```python
from build123d import *

# Parameters (mm, degrees)
ESBO_O1_R                = 7.5
RESSALTO_EXTRUS_O1_DEPTH = 1.2
ESBO_O2_R                = 3
RESSALTO_EXTRUS_O2_DEPTH = 7.2
ESBO_O3_R                = 4
RESSALTO_EXTRUS_O3_DEPTH = 1
ESBO_O4_R                = 3.25
ESBO_O4_R_2              = 3.0000000000000004
CORTE_EXTRUS_O1_DEPTH    = 0.5
ESBO_O5_R                = 2.5
CORTE_EXTRUS_O4_DEPTH    = 1
FILETE1_R                = 0.5


with BuildPart() as part:
    # Esboço1 → Ressalto-extrusão1 (new body)
    with BuildSketch(Plane(origin=(0, 0, 0), x_dir=(1, 0, 0), z_dir=(0, 1, 0))):
        with Locations(Location((0, 0, 0), (0, 0, 270))):
            Circle(ESBO_O1_R)
    extrude(amount=RESSALTO_EXTRUS_O1_DEPTH)

    # Esboço2 → Ressalto-extrusão2 (add)
    with BuildSketch(Plane.XZ):
        with Locations(Location((0, 0, 0), (0, 0, 90))):
            Circle(ESBO_O2_R)
    extrude(amount=RESSALTO_EXTRUS_O2_DEPTH)

    # Esboço3 → Ressalto-extrusão3 (add)
    with BuildSketch(Plane.XZ.offset(7.2)):
        with Locations(Location((0, 0, 0), (0, 0, 270))):
            Circle(ESBO_O3_R)
    extrude(amount=-RESSALTO_EXTRUS_O3_DEPTH)

    # Esboço4 → Corte-extrusão1 (cut)
    with BuildSketch(Plane(origin=(0, -6.2, 0), x_dir=(1, 0, 0), z_dir=(0, 1, 0))):
        with Locations(Location((0, 0, 0), (0, 0, 270))):
            Circle(ESBO_O4_R)
        with Locations(Location((0, 0, 0), (0, 0, 270))):
            Circle(ESBO_O4_R_2, mode=Mode.SUBTRACT)
    extrude(amount=-CORTE_EXTRUS_O1_DEPTH, mode=Mode.SUBTRACT)

    # Esboço5 → Corte-extrusão4 (cut)
    with BuildSketch(Plane.XZ.offset(7.2)):
        with Locations(Location((0, 0, 0), (0, 0, 270))):
            Circle(ESBO_O5_R)
    extrude(amount=-CORTE_EXTRUS_O4_DEPTH, mode=Mode.SUBTRACT)

    # Filete1
    # the kernel refuses this fillet: 0.5 mm, written as the material it adds along each edge
    with BuildSketch(Plane(origin=(0, -6.7, 0), x_dir=(-1.8e-16, 0, 1), z_dir=(-1, 0, -1.8e-16))) as filete1_piece_1:
        with BuildLine():
            CenterArc((3.5000000000000004, 0.4330127018922436), FILETE1_R, 180, 60.000000000001364)
            Line((3.2500000000000107, 1.865e-14), (3.0000000000000004, 0))
            Line((3.0000000000000004, 0), (3.0000000000000004, 0.4330127018922436))
        make_face()
    revolve(axis=Axis((0, -6.7, 0), (0, 1, 0)))
    with BuildSketch(Plane(origin=(0, -6.2, 0), x_dir=(-1.8e-16, 0, -1), z_dir=(-1, 0, 1.8e-16))) as filete1_piece_2:
        with BuildLine():
            CenterArc((2.5 - FILETE1_R, FILETE1_R), FILETE1_R, 270, 90)
            Line((2.5 - FILETE1_R, 0), (2.5, 0))
            Line((2.5, 0), (2.5, FILETE1_R))
        make_face()
    revolve(axis=Axis((0, -6.2, 0), (0, -1, 0)))
    # the kernel refuses this fillet: 0.5 mm, written as the material it takes off along each edge
    with BuildSketch(Plane(origin=(0, -7.2, 0), x_dir=(-1.8e-16, 0, -1), z_dir=(-1, 0, 1.8e-16))) as filete1_2_piece_1:
        with BuildLine():
            CenterArc((4 - FILETE1_R, -FILETE1_R), FILETE1_R, 0, 90)
            Line((4 - FILETE1_R, 0), (4, 0))
            Line((4, 0), (4, -FILETE1_R))
        make_face()
    revolve(axis=Axis((0, -7.2, 0), (0, -1, 0)), mode=Mode.SUBTRACT)
    with BuildSketch(Plane(origin=(0, -6.2, 0), x_dir=(-1.8e-16, 0, 1), z_dir=(-1, 0, -1.8e-16))) as filete1_2_piece_2:
        with BuildLine():
            CenterArc((3.25 + FILETE1_R, -FILETE1_R), FILETE1_R, 90, 90)
            Line((3.25 + FILETE1_R, 0), (3.25, 0))
            Line((3.25, 0), (3.25, -FILETE1_R))
        make_face()
    revolve(axis=Axis((0, -6.2, 0), (0, 1, 0)), mode=Mode.SUBTRACT)
    with BuildSketch(Plane(origin=(0, -7.2, 0), x_dir=(-1.8e-16, 0, -1), z_dir=(-1, 0, 1.8e-16))) as filete1_2_piece_3:
        with BuildLine():
            CenterArc((2.5 + FILETE1_R, -FILETE1_R), FILETE1_R, 90, 90)
            Line((2.5, -FILETE1_R), (2.5, 0))
            Line((2.5, 0), (2.5 + FILETE1_R, 0))
        make_face()
    revolve(axis=Axis((0, -7.2, 0), (0, -1, 0)), mode=Mode.SUBTRACT)


solid = part.part
```
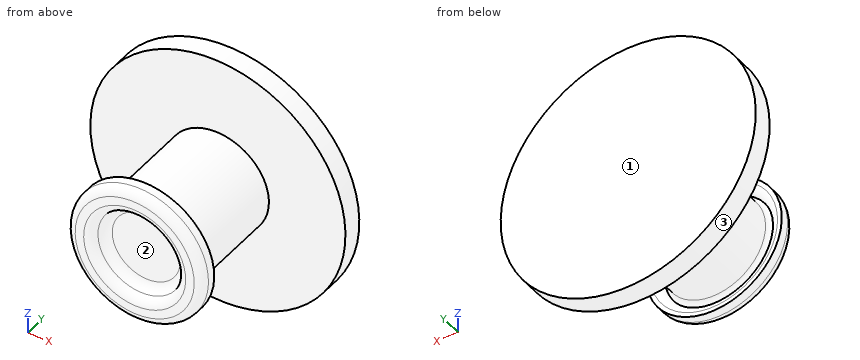
Part model, mm, in its own coordinate system. Face numbers are marked on the shaded views. Round coordinates to 2 decimals unless told otherwise and drop trailing zeros. Write each loop counter-clockwise with the first axis right and the second up, starting at its lowest first coordinate (ties: lowest second). Pieces come first, ordered by that corner, then holes. Notation, with made-up numbers: M 49.5,85 L 88.5,85 A30 cw 88.5,112 Z; hole C -12.75,-38 d9. An arc over 180 degrees is marked long. Answer as CSV lines item,"result". Start each with the question number.
1) Band-saw the part on C-C (z = -5.75). List the corners of the cut face in (x, y), then the cut area to 3 significant figures.
2) Mould opens along Z. For the marked faces 1, 2 and 3 say: +Z half, -Z half, draft (parallel to the pull), parting line (faces both ways), or undercut.
3) Drop flat-ended pins along their axis: pin 1 (2 mm diameter, centred on y = -5.5, z = 2.5, fed in from +X); pin 2 (2 mm diameter, centred on x = -0.5, z = -1, fed in from -Y). Give the stop position or say it passes through.
4) Band-saw the part on D-D (y = 0.25). List the corners of the cut face in (x, z).
5) Band-saw the part on A-A (x = -4.5). List the corners of the cut face in (y, z).
6) Band-saw the part on B-B (y = -4). List the corners of the cut face in (x, z), then the cut area to 3 significant figures.
7) Drill centre lines: L1, parallel to Y at x = -3.5, z = -5.25; L2, parallel to Y at x = 1.25, z = 1.25; L3, parallel to Z at x = 6, y = 0.25. Where is each one in solid material? Low to high.
Worked out:
1,outline,"M -4.82,0 L 4.82,0 L 4.82,1.2 L -4.82,1.2 Z"
1,area,"11.6 mm²"
2,face 1,"draft"
2,face 2,"undercut"
2,face 3,"parting line"
3,pin 1,"x = 3.58"
3,pin 2,"y = -6.21"
4,outline,"C 0,0 d15"
5,outline,"M 0,-6 L 1.2,-6 L 1.2,6 L 0,6 Z"
6,outline,"C 0,0 d6"
6,area,"28.3 mm²"
7,L1,"0 to 1.2"
7,L2,"-6.2 to 1.2"
7,L3,"-4.5 to 4.5"
